The listing builds one solid part. Answer for the finished solid, in the listing's coordinates (mm). Round coordinates to 2 decimals unless told otherwise and drop trailing zeros. Loops run counter-clockwise (first coordinate to the right, second up) from the corner with the lowest first, then second, coordinate; pieces in that order, holes last. Notation, with made-up numbers: (-2.5, -37.5) - (44.5, -37.5) arc R37 ccw to (44.5, -0.5) - close; hole circle Ø5 at (-12.75, 75). An arc over 180 degrees is marked (long way). One line per item, written item: value.
Autodesk Inventor part; units mm, degrees
ref_plane "YZ Plane" through (0, 0, 0) normal (1, 0, 0) x (0, 1, 0)
ref_plane "XZ Plane" through (0, 0, 0) normal (0, 1, 0) x (-1, 0, 0)
ref_plane "XY Plane" through (0, 0, 0) normal (0, 0, 1) x (1, 0, 0)
sketch "Sketch1" plane through (0, 0, 0) normal (0, 0, 1) x (1, 0, 0)
  line L0 (0, 0) -> (444.5, 0)
  line L1 (444.5, 0) -> (444.5, 127)
  line L2 (444.5, 127) -> (0, 127)
  line L3 (0, 127) -> (0, 0)
  dimension "d0" = 444.5
  dimension "d1" = 127
extrude "Extrusion1" add sketch "Sketch1" along normal blind 6.35
sketch "Sketch2" plane through (0, 0, 6.35) normal (0, 0, 1) x (1, 0, 0)
  line L0 (0, 0) -> (444.5, 0)
  line L1 (38.0923, 0) -> (0, 38.0919)
  line L2 (0, 127) -> (0, 0)
  line L3 (0, 0) -> (444.5, 0)
  line L4 (444.5, 0) -> (444.5, 127)
  line L5 (444.5, 0) -> (406.4, 0)
  line L6 (444.5, 0) -> (482.6, 0) construction
  line L7 (444.5, 0) -> (444.5, 38.0919)
  line L8 (444.5, 38.0919) -> (406.4086, 0)
  point P0 (419.1126, 0)
  dimension "d19" = 38.1
  dimension "d20" = 180
extrude "Extrusion2" cut sketch "Sketch2" against normal blind 50.8
sketch "Sketch3" plane through (0, 0, 6.35) normal (0, 0, 1) x (1, 0, 0)
  line L0 (0, 77.664) -> (80.645, 77.664) construction
  line L1 (444.5, 127) -> (0, 127)
  line L2 (80.645, 127) -> (161.29, 127) construction
  circle A0 centre (80.645, 46.355) radius 14.2748
  line L3 (444.5, 38.0919) -> (444.5, 127)
  line L4 (444.5, 77.664) -> (525.145, 77.664) construction
  line L5 (444.5, 38.0919) -> (444.5, 127)
  line L6 (444.5, 46.355) -> (525.145, 46.355) construction
  circle A1 centre (363.855, 46.355) radius 14.2748
  line L7 (444.5, 127) -> (0, 127)
  line L8 (0, 127) -> (0, 38.0919)
  circle A2 centre (181.483, 46.355) radius 21.59
  circle A3 centre (263.017, 46.355) radius 21.59
  line L9 (181.483, 46.355) -> (205.486, 46.355)
  line L10 (205.486, 46.355) -> (205.486, 53.3654)
  circle A4 centre (205.486, 53.3654) radius 1.7526
  line L11 (205.486, 46.355) -> (205.486, 39.3446)
  circle A5 centre (205.486, 39.3446) radius 1.7526
  line L12 (181.483, 46.355) -> (157.48, 46.355)
  line L13 (157.48, 46.355) -> (157.48, 53.3654)
  line L14 (157.48, 46.355) -> (157.48, 39.3446)
  circle A6 centre (157.48, 39.3446) radius 1.7526
  circle A7 centre (157.48, 53.3654) radius 1.7526
  line L15 (263.017, 46.355) -> (287.02, 46.355)
  line L16 (263.017, 46.355) -> (239.014, 46.355)
  line L17 (239.014, 46.355) -> (239.014, 53.3654)
  line L18 (239.014, 46.355) -> (239.014, 39.3446)
  line L19 (287.02, 46.355) -> (287.02, 39.3446)
  line L20 (287.02, 46.355) -> (287.02, 53.3654)
  circle A8 centre (287.02, 53.3654) radius 1.7526
  circle A9 centre (287.02, 39.3446) radius 1.7526
  circle A10 centre (239.014, 39.3446) radius 1.7526
  circle A11 centre (239.014, 53.3654) radius 1.7526
  line L21 (263.017, 46.355) -> (256.667, 46.355)
  line L22 (406.4086, 0) -> (444.5, 38.0919)
  line L23 (444.5, 38.0919) -> (444.5, 127)
  line L24 (444.5, 127) -> (0, 127)
  line L25 (0, 127) -> (0, 38.0919)
  line L26 (0, 38.0919) -> (38.0923, 0)
  line L27 (38.0923, 0) -> (406.4086, 0)
  line L28 (406.4086, 0) -> (444.5, 38.0919)
  line L29 (444.5, 38.0919) -> (444.5, 127)
  line L30 (444.5, 127) -> (0, 127)
  line L31 (0, 127) -> (0, 38.0919)
  line L32 (0, 38.0919) -> (38.0923, 0)
  line L33 (38.0923, 0) -> (406.4086, 0)
  line L34 (38.0923, 0) -> (0, 38.0919)
  line L35 (0, 38.0919) -> (0, 127)
  line L36 (0, 127) -> (444.5, 127)
  line L37 (444.5, 127) -> (444.5, 38.0919)
  line L38 (444.5, 38.0919) -> (406.4086, 0)
  line L39 (406.4086, 0) -> (38.0923, 0)
  point P0 (0, 0)
  dimension "d10" = 28.5496
  dimension "d18" = 28.5496
  dimension "d31" = 43.18
  dimension "d32" = 43.18
  dimension "d55" = 24.003
  dimension "d56" = 7.0104
  dimension "d57" = 3.5052
  dimension "d58" = 7.0104
  dimension "d59" = 3.5052
  dimension "d60" = 24.003
  dimension "d61" = 7.0104
  dimension "d62" = 7.0104
  dimension "d63" = 3.5052
  dimension "d64" = 3.5052
  dimension "d65" = 24.003
  dimension "d66" = 24.003
  dimension "d67" = 3.5052
  dimension "d68" = 3.5052
  dimension "d69" = 3.5052
  dimension "d70" = 3.5052
  dimension "d73" = 6.35
  dimension "d74" = 181.483
  dimension "d75" = 181.483
extrude "Extrusion3" cut sketch "Sketch3" against normal blind 50.8 contours A0 | A1
extrude "Extrusion4" cut sketch "Sketch3" against normal blind 25.4 contours L9 L12 A2 | A2 L12 L9 | L15 L16 A3 | A3 L16 L15
thicken "Thicken1" operation add thickness 20.828 both sides no extend neighbours yes toward (0, 1, 0) faces at (160.8644, 0, 2.1167)
extrude "Extrusion6" cut sketch "Sketch3" against normal blind 25.4 contours A4 | A5 | A6 | A7 | A8 | A9 | A10 | A11
properties part number "MecanumDriveTrainPlate17-18"
1) This flat-tipped pin is pushed along its axis until it touches: pin 1 Ø1 at (y, z) = (32.5, 4) entering from +X. Where does it stop, or does it pass through?
Final values:
pin 1: x = 439.41
2) Consider L1, parallel to Y at x = 287.02, z = 3.25; L2, parallel to X at y = 31.5, z = 4.25; L3, parallel to X at y = 26.5, z = 3.5. Determine where each line is inside the solid, lowest interval first.
Final values:
L1: 20.83 to 37.59, 41.1 to 51.61, 55.12 to 127
L2: 6.59 to 165.82, 197.15 to 247.35, 278.68 to 437.91
L3: 11.59 to 173, 189.96 to 254.54, 271.5 to 432.91
3) For a pull along X with two mould halves and no side action, classify faces 1 (the cylindrical face through (159.914, 47.304, 3.219)), 2 (the flat face through (435.99, 29.58, 3.22)), 3 (the flat face through (219, 75, 6.35)) as released by +X, released by -X, zero draft, split by the parting line, or undercut.
Final values:
face 1: undercut
face 2: released by +X
face 3: zero draft
4) A cutting plane is placed at B-B on z = 4.75. Give the number of separate pieces and of enclosed holes in the cut face, and give its area (3 significant figures).
Final values:
separate pieces: 1
enclosed holes: 12
area: 42,600 mm2
5) A cutting plane is placed at A-A on x = 367. Give the vertices of the cut face in (y, z).
Final values:
outline: (20.83, 0) - (32.43, 0) - (32.43, 6.35) - (20.83, 6.35) - close; (60.28, 0) - (127, 0) - (127, 6.35) - (60.28, 6.35) - close
